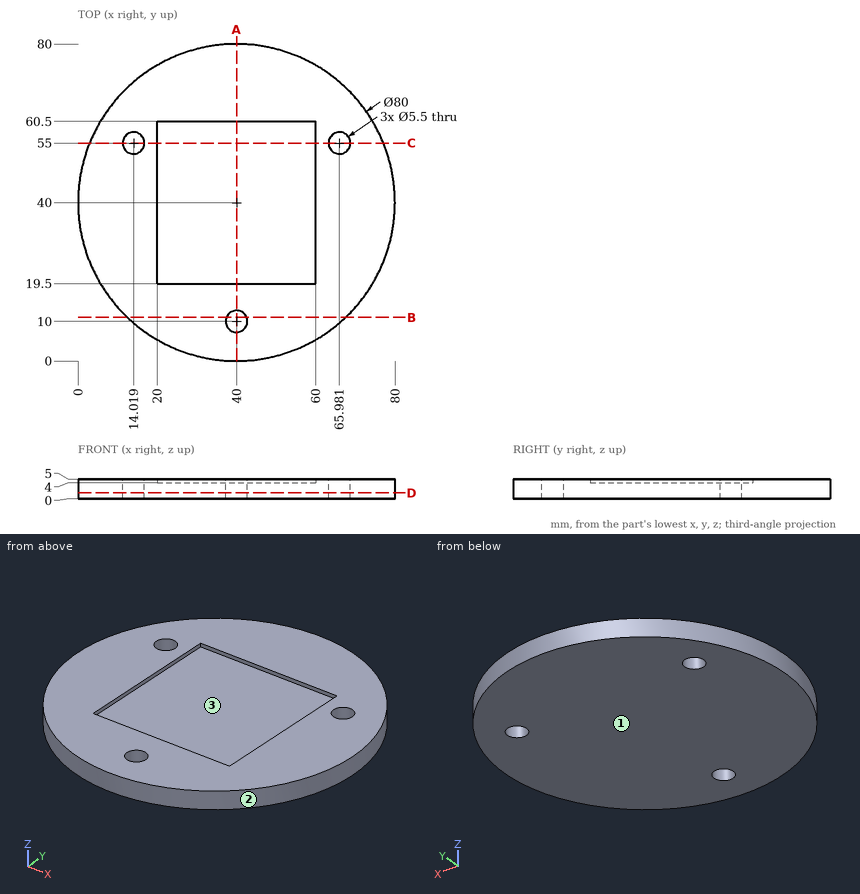
For this review, use the dimensioned drawing (mm, ordinates from the lowest corner) and the shaded views. Round coordinates to 2 decimals unless told otherwise and drop trailing zeros. Order: outer loops, then holes, each group sorted by start corner. A loop starts at its lowest first (then second) coordinate and runs counter-clockwise, first axis right, second up. Notation, with made-up numbers: M 43,76 L 79,76 A25 cw 79,112 Z; hole C 62.5,73.25 d11. An arc over 180 degrees is marked long. Use a Markdown table: item, result. Add a question column.
Item 1: Add section C-C, the plane y = 55. Give the boundary of the cut face in (x, z), then the cut area to 3 significant figures.
Item 2: Add section D-D, the plane z = 1.5. Give the boundary of the cut face in (x, y), then the cut area to 3 significant figures.
Item 3: Insertion check: pin 1 (0.8 mm diameter, centred on x = 42.5, z = 4.5, fed in from +Y) (3 decimals); pin 2 (0.8 mm diameter, centred on x = 34.5, z = 4.5, fed in from -Y); pin 3 (1.1 mm diameter, centred on y = 42.5, z = 4.5, fed in from -X). Each pin has a flat end and moves straight along its axis. Give the tip position at first contact, or say it passes through.
Item 4: To check wall thickness, follow line 1 along Y through (x, z) = (40, 1); line 2 along X through (y, z) = (40.5, 4.25); line 3 along Z through (x, y) = (43, 45). State the ranges of each line that lie inside material, in increasing order.
Item 5: Add section B-B, the plane y = 11. Give the boundary of the cut face in (x, z), then the cut area to 3 significant figures.
Item 6: Add section A-A, the plane x = 40. Give the boundary of the cut face in (y, z).
Item 7: Mouldability with a two-part tool opening along X and no side actions: class the marked faces 1, 2 and 3 as released by +X, released by -X, zero draft, split by the parting line, or undercut.
Geometry results:
| question | item | result |
|---|---|---|
| 1 | outline | M 2.92,0 L 11.27,0 L 11.27,5 L 2.92,5 Z; M 16.77,0 L 63.23,0 L 63.23,5 L 60,5 L 60,4 L 20,4 L 20,5 L 16.77,5 Z; M 68.73,0 L 77.08,0 L 77.08,5 L 68.73,5 Z |
| 1 | area | 276 mm² |
| 2 | outline | C 40,40 d80; hole C 14.02,55 d5.5; hole C 40,10 d5.5; hole C 65.98,55 d5.5 |
| 2 | area | 4,960 mm² |
| 3 | pin 1 | stops at y = 79.945 |
| 3 | pin 2 | stops at y = 0.33 |
| 3 | pin 3 | stops at x = 0.05 |
| 4 | line 1 | y = 0 to 7.25, 12.75 to 80 |
| 4 | line 2 | x = 0 to 20, 60 to 80 |
| 4 | line 3 | z = 0 to 4 |
| 5 | outline | M 12.45,0 L 37.44,0 L 37.44,5 L 12.45,5 Z; M 42.56,0 L 67.55,0 L 67.55,5 L 42.56,5 Z |
| 5 | area | 250 mm² |
| 6 | outline | M 0,0 L 7.25,0 L 7.25,5 L 0,5 Z; M 12.75,0 L 80,0 L 80,5 L 60.5,5 L 60.5,4 L 19.5,4 L 19.5,5 L 12.75,5 Z |
| 7 | face 1 | zero draft |
| 7 | face 2 | split by the parting line |
| 7 | face 3 | undercut |
